```python
from build123d import *

# Parameters (mm, degrees)
F0_W     = 70
F0_H     = 120
F1_DEPTH = 4
F2_R     = 5
F3_R     = 10.25
F4_DEPTH = 25
F5_W     = 50
F5_H     = 11
F6_DEPTH = 25
F7_R     = 1


with BuildPart() as f1:
    # F0 (on Front) → F1 (new body)
    with BuildSketch(Plane.XZ):
        Rectangle(F0_W, F0_H)
        with BuildLine():
            ThreePointArc((-29, 51.5), (-30.767766953, 55.767766953), (-26.5, 54))
            Line((-26.5, 54), (26.5, 54))
            ThreePointArc((26.5, 54), (29, 56.5), (31.5, 54))
            ThreePointArc((31.5, 54), (30.767766953, 52.232233047), (29, 51.5))
            Line((29, 51.5), (29, -51.5))
            ThreePointArc((29, -51.5), (30.767766953, -52.232233047), (31.5, -54))
            ThreePointArc((31.5, -54), (29, -56.5), (26.5, -54))
            Line((26.5, -54), (-26.5, -54))
            ThreePointArc((-26.5, -54), (-30.767766953, -55.767766953), (-29, -51.5))
            Line((-29, -51.5), (-29, 51.5))
        make_face(mode=Mode.SUBTRACT)
        with BuildLine():
            Line((26.5, 54), (-26.5, 54))
            ThreePointArc((-26.5, 54), (-27.232233047, 52.232233047), (-29, 51.5))
            Line((-29, 51.5), (-29, -51.5))
            ThreePointArc((-29, -51.5), (-27.232233047, -52.232233047), (-26.5, -54))
            Line((-26.5, -54), (26.5, -54))
            ThreePointArc((26.5, -54), (27.232233047, -52.232233047), (29, -51.5))
            Line((29, -51.5), (29, 51.5))
            ThreePointArc((29, 51.5), (27.232233047, 52.232233047), (26.5, 54))
        make_face()
    extrude(amount=F1_DEPTH)

    # F2
    f2_edges = [f1.edges().sort_by_distance(p)[0] for p in [
        (-35, -2, 60),
        (35, -2, 60),
        (-35, -2, -60),
        (35, -2, -60),
    ]]
    fillet(f2_edges, radius=F2_R)

    # F3 (on face) → F4 (cut)
    with BuildSketch(Plane.XZ.offset(4)):
        with Locations((15, 30)):
            Circle(F3_R)
    extrude(amount=-F4_DEPTH, mode=Mode.SUBTRACT)

    # F5 (on face) → F6 (cut)
    with BuildSketch(Plane.XZ.offset(4)):
        with Locations((0, -37.5)):
            Rectangle(F5_W, F5_H)
    extrude(amount=-F6_DEPTH, mode=Mode.SUBTRACT)

    # F7
    f7_edges = [f1.edges().sort_by_distance(p)[0] for p in [
        (-25, -2, -43),
        (-25, -2, -32),
        (25, -2, -32),
        (25, -2, -43),
    ]]
    fillet(f7_edges, radius=F7_R)


solid = f1.part
```
Verification items for the finished model (mm, model axes). A direction names the side the tool comes from. Coordinates: 2 decimals unless noted, no trailing zeros. Loops run counter-clockwise (first coordinate to the right, second up) from the corner with the lowest first, then second, coordinate; pieces in that order, holes last. Notation, with made-up numbers: (-4.75, 89.5) - (4.25, 89.5) arc R24 ccw to (4.25, 127.5) - close; hole circle Ø10 at (17.5, 13). An arc over 180 degrees is marked (long way). Return JSON: item names as keys, results as strings.
1. Mould release check, pull along X, two halves, no side actions. Record for faces 3 (the flat face through (0, -2, -32)), 4 (the flat face through (35, -2, -1)), 5 (the flat face through (-35, -2, -1)): +X half, -X half, draft (parallel to the pull), parting line (faces both ways), or undercut.
Established:
{"face 3": "undercut", "face 4": "+X half", "face 5": "-X half"}
2. Section check A-A, the plane x = 15. Record the boundary of the cut face in (y, z), then the cut area to 3 significant figures.
Established:
{"outline": "(-4, -60) - (0, -60) - (0, -43) - (-4, -43) - close; (-4, -32) - (0, -32) - (0, 19.75) - (-4, 19.75) - close; (-4, 40.25) - (0, 40.25) - (0, 60) - (-4, 60) - close", "area": "354 mm2"}
3. Tool access check on faces 1 (the flat face through (0, -2, -43)), 2 (the flat face through (0, -2, 60)). Record the directions out of +Z, -Z, +X, -X, +Y, -Y that give a thin tool (end or side, any length) a straight path to the whole face; none if there is none.
Established:
{"face 1": "+Y, -Y", "face 2": "+Z, +X, -X, +Y, -Y"}
4. Section check C-C, the plane y = -2.35. Record the boundary of the cut face in (x, z), then the cut area to 3 significant figures.
Established:
{"outline": "(-35, -55) arc R5 ccw to (-30, -60) - (30, -60) arc R5 ccw to (35, -55) - (35, 55) arc R5 ccw to (30, 60) - (-30, 60) arc R5 ccw to (-35, 55) - close; hole circle Ø5 at (-29, -54); hole circle Ø5 at (-29, 54); hole (-25, -42) arc R1 ccw to (-24, -43) - (24, -43) arc R1 ccw to (25, -42) - (25, -33) arc R1 ccw to (24, -32) - (-24, -32) arc R1 ccw to (-25, -33) - close; hole circle Ø20.5 at (15, 30); hole circle Ø5 at (29, -54); hole circle Ø5 at (29, 54)", "area": "7,420 mm2"}
5. Thickness scan on L1, parallel to X at y = -1.2, z = 54; L2, parallel to Z at x = 15, y = -3.2; L3, parallel to Z at x = -28, y = -2.8. Record the ranges inside material, lowest first.
Established:
{"L1": "x = -35 to -31.5, -26.5 to 26.5, 31.5 to 35", "L2": "z = -60 to -43, -32 to 19.75, 40.25 to 60", "L3": "z = -60 to -56.29, -51.71 to 51.71, 56.29 to 60"}
6. Section check B-B, the plane z = 30. Record the boundary of the cut face in (x, y), then the cut area to 3 significant figures.
Established:
{"outline": "(-35, -4) - (4.75, -4) - (4.75, 0) - (-35, 0) - close; (25.25, -4) - (35, -4) - (35, 0) - (25.25, 0) - close", "area": "198 mm2"}
